Autodesk Inventor part; units mm, degrees
ref_plane "YZ Plane" through (0, 0, 0) normal (1, 0, 0) x (0, 1, 0)
ref_plane "XZ Plane" through (0, 0, 0) normal (0, 1, 0) x (-1, 0, 0)
ref_plane "XY Plane" through (0, 0, 0) normal (0, 0, 1) x (1, 0, 0)
sketch "Schizzo1" plane through (0, 0, 0) normal (0, 1, 0) x (-1, 0, 0)
  circle A0 centre (0, 0) radius 95
  circle A1 centre (0, 0) radius 45.25
  circle A2 centre (0, 0) radius 75 construction
  circle A3 centre (0, 75) radius 9
  circle A4 centre (-75, 0) radius 9
  circle A5 centre (0, -75) radius 9
  circle A6 centre (75, 0) radius 9
  dimension "d2" = 150
  dimension "d0" = 190
  dimension "d1" = 90.5
  dimension "d3" = 18
  dimension "d6" = 360
extrude "Estrusione1" add sketch "Schizzo1" along normal blind 18
properties part number "06-01-2023 flangia DN80"
Geometry check sheet. Reference: the model listing, model coordinates, mm. Round coordinates to 2 decimals unless told otherwise and drop trailing zeros. Loops run counter-clockwise (first coordinate to the right, second up) from the corner with the lowest first, then second, coordinate; pieces in that order, holes last. Notation, with made-up numbers: (82, 68) - (134, 68) arc R28 ccw to (134, 86) - close; hole circle Ø8 at (22.5, 70.5). An arc over 180 degrees is marked (long way). One line per question, with ' | ' between items. Start each with the question number.
1. Cross-section at D-D on x = -37. Record the cut outline in (y, z), then the cut area to 3 significant figures.
2. Scan lines: line 1 (Z direction, x = 0, y = 8); line 2 (Z direction, x = -5, y = 15.75); line 3 (Z direction, x = -77.5, y = 6.5). Record each from-to range of solid material in increasing order. Write a range as [from, to].
3. Cross-section at A-A on z = 0. Record the cut outline in (x, y), then the cut area to 3 significant figures.
4. Depth check by flat-ended pin: pin 1 (5 mm diameter, centred on x = 28, z = 68, fed in from -Y); pin 2 (4 mm diameter, centred on x = 74, y = 3.5, fed in from +Z); pin 3 (8 mm diameter, centred on y = 8, z = -25.5, fed in from +X); pin 4 (16 mm diameter, centred on x = 0, z = -75, fed in from -Y). Enter the tip coordinate at first touch or a pass-through.
5. Cross-section at B-B on x = 0. Record the cut outline in (y, z).
6. Cross-section at C-C on y = 7. Record the cut outline in (x, z), then the cut area to 3 significant figures.
7. Draft check along X on faces 1 (the face through (-41, 18, -20)), 2 (the face through (20.59, 8.87, 92.74)), 3 (the face through (-43.16, 8.87, -13.59)). Enter one of: released by +X, released by -X, zero draft, split by the parting line, or undercut.
Taken from the geometry:
1) outline: (0, -87.5) - (18, -87.5) - (18, -26.05) - (0, -26.05) - close; (0, 26.05) - (18, 26.05) - (18, 87.5) - (0, 87.5) - close | area: 2,210 mm²
2) line 1: [-95, -84], [-66, -45.25], [45.25, 66], [84, 95] | line 2: [-94.87, -82.48], [-67.52, -44.97], [44.97, 67.52], [82.48, 94.87] | line 3: [-54.94, -8.65], [8.65, 54.94]
3) outline: (-95, 0) - (-84, 0) - (-84, 18) - (-95, 18) - close; (-66, 0) - (-45.25, 0) - (-45.25, 18) - (-66, 18) - close; (45.25, 0) - (66, 0) - (66, 18) - (45.25, 18) - close; (84, 0) - (95, 0) - (95, 18) - (84, 18) - close | area: 1,140 mm²
4) pin 1: y = 0 | pin 2: z = 61.98 | pin 3: x = 92.54 | pin 4: through
5) outline: (0, -95) - (18, -95) - (18, -84) - (0, -84) - close; (0, -66) - (18, -66) - (18, -45.25) - (0, -45.25) - close; (0, 45.25) - (18, 45.25) - (18, 66) - (0, 66) - close; (0, 84) - (18, 84) - (18, 95) - (0, 95) - close
6) outline: circle Ø190 at (0, 0); hole circle Ø18 at (-75, 0); hole circle Ø90.5 at (0, 0); hole circle Ø18 at (0, -75); hole circle Ø18 at (0, 75); hole circle Ø18 at (75, 0) | area: 20,900 mm²
7) face 1: zero draft | face 2: split by the parting line | face 3: undercut
